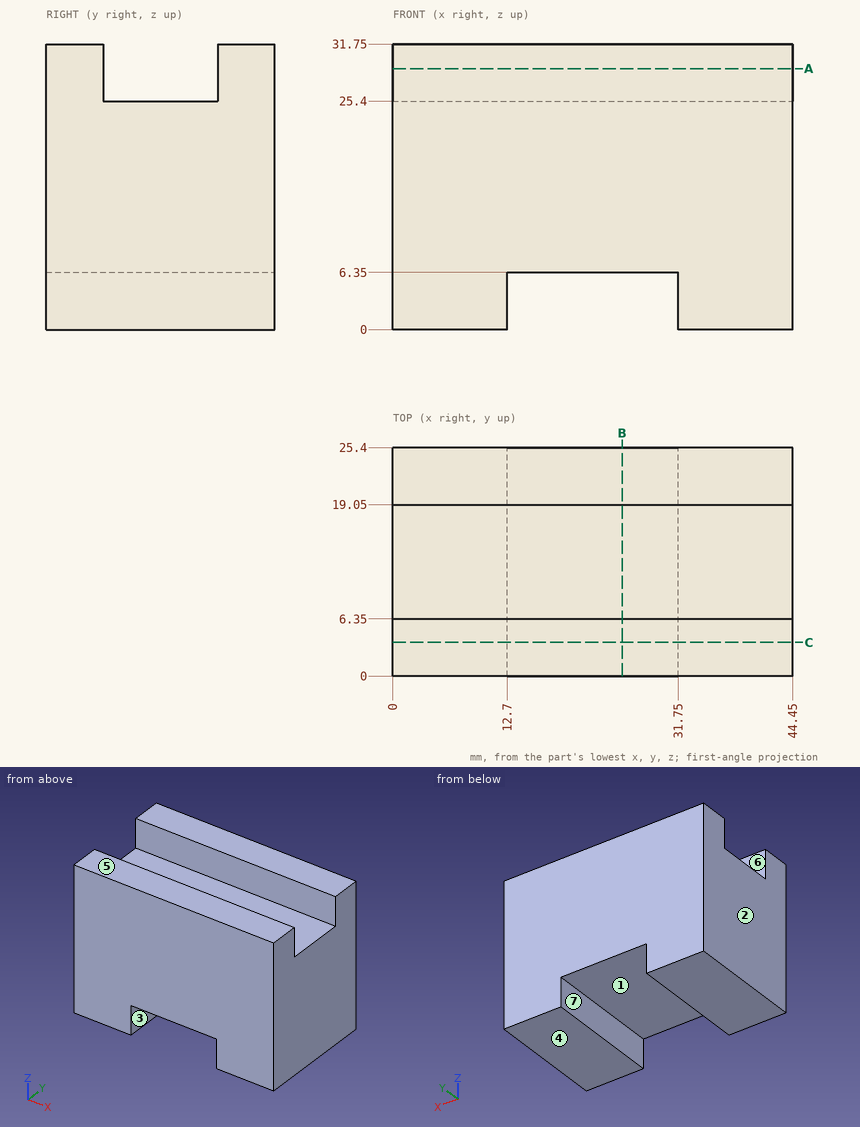
Can you work these out from the drawing? Everything is in mm from the part's minimum corner. A direction names the side the tool comes from. Give positions to 0.01 mm unless a question says otherwise; leave off trailing zeros. Order: outer loops, then holes, each group sorted by start corner. A loop starts at its lowest first (then second) coordinate and runs counter-clockwise, first axis right, second up. Notation, with made-up numbers: (37.25, -26) -> (46.25, -26) arc R16 cw to (46.25, -18) -> close; hole circle Ø10 at (33, -25.5). An arc over 180 degrees is marked (long way). Return JSON: item names as keys, results as strings.
1. Imagine slicing it at A-A on z = 29. List the corners of the cut face in (x, y) for me, then the cut area to 3 significant figures.
Answer list:
{"outline": "(0, 0) -> (44.45, 0) -> (44.45, 6.35) -> (0, 6.35) -> close; (0, 19.05) -> (44.45, 19.05) -> (44.45, 25.4) -> (0, 25.4) -> close", "area": "565 mm2"}
2. Thinking about a two-plate mould opening in X: for the marked faces 1, 2, 3 and 4, which applies, pulls with the +X half, pulls with the -X half, needs draft (parallel to the pull), parting line crosses it, or undercut?
Answer list:
{"face 1": "undercut", "face 2": "pulls with the -X half", "face 3": "undercut", "face 4": "needs draft"}
3. For pin 1 Ø4 at (x, y) = (29.5, 12) entering from +Z; pin 2 Ø15 at (x, y) = (22.5, 7.5) entering from -Z, each with a flat end and sliding along its axis, tell me the tip position at first contact or that it passes through.
Answer list:
{"pin 1": "stops at z = 25.4", "pin 2": "stops at z = 6.35"}
4. Imagine slicing it at C-C on y = 3.75. List the corners of the cut face in (x, z) for me, then the cut area to 3 significant figures.
Answer list:
{"outline": "(0, 0) -> (12.7, 0) -> (12.7, 6.35) -> (31.75, 6.35) -> (31.75, 0) -> (44.45, 0) -> (44.45, 31.75) -> (0, 31.75) -> close", "area": "1,290 mm2"}
5. Imagine slicing it at B-B on x = 25.5. List the corners of the cut face in (y, z) for me, then the cut area to 3 significant figures.
Answer list:
{"outline": "(0, 6.35) -> (25.4, 6.35) -> (25.4, 31.75) -> (19.05, 31.75) -> (19.05, 25.4) -> (6.35, 25.4) -> (6.35, 31.75) -> (0, 31.75) -> close", "area": "565 mm2"}
6. I need wall thicknesses on line 1 (X direction, y = 1.5, z = 5.5); line 2 (Z direction, x = 26, y = 20); line 3 (Z direction, x = 31, y = 17.75). Which ranges of each line are inside material? Lowest first, please. Write a range as from..to.
Answer list:
{"line 1": "x = 0..12.7, 31.75..44.45", "line 2": "z = 6.35..31.75", "line 3": "z = 6.35..25.4"}
7. On a 3-axis mill with a long thin cutter (end or side, diameter ignored), from which of +Z, -Z, +X, -X, +Y, -Y can I reach the whole of each face in a straight line? I mean the marked faces 5, 6 and 7. Say none if no direction works.
Answer list:
{"face 5": "+Z, +X, -X, +Y, -Y", "face 6": "+Z, +X, -X", "face 7": "-Z, +Y, -Y"}
